The drawing under review shows one solid part. Ordinate dimensions are in mm from its lowest x, y, z. Coordinates: 2 decimals unless noted, no trailing zeros. Write each loop counter-clockwise with the first axis right and the second up, starting at its lowest first coordinate (ties: lowest second). Pieces come first, ordered by that corner, then holes. Notation, with made-up numbers: (61, -30.75) - (93, -30.75) arc R9 cw to (93, -15.75) - close; hole circle Ø10 at (7.25, 71). An arc over 180 degrees is marked (long way). Use a Markdown table: item, result.
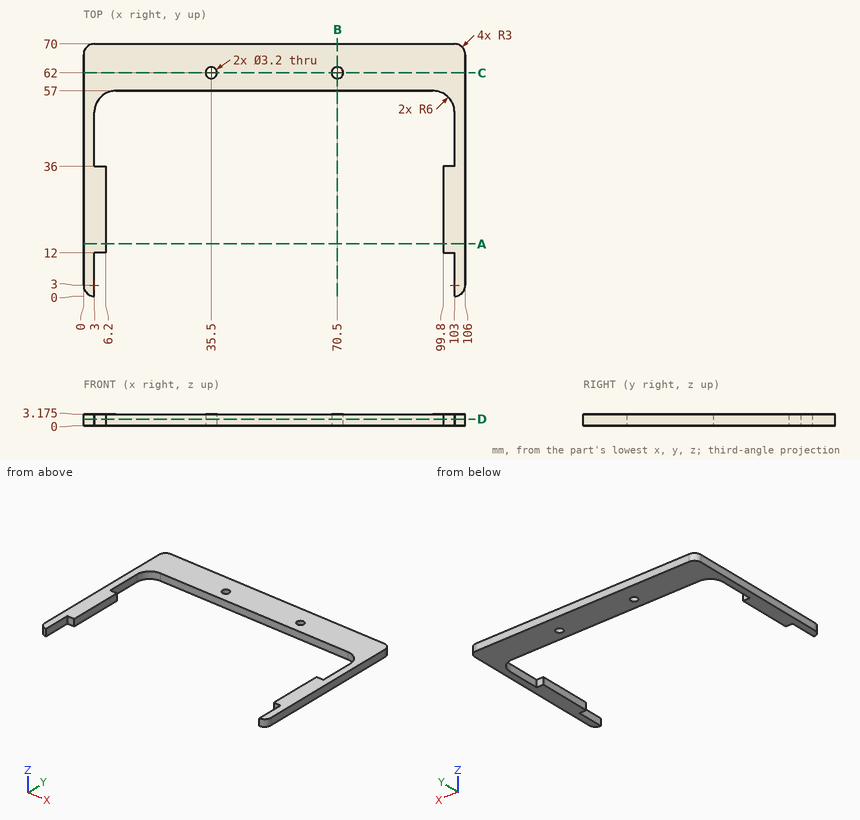
(1) Take a section at A-A on y = 14.5. Write out the cut boundary in (x, z) (3 decimals), and give its area (3 significant figures).
Determined:
| item | result |
|---|---|
| outline | (0, 0) - (6.2, 0) - (6.2, 3.175) - (0, 3.175) - close; (99.8, 0) - (106, 0) - (106, 3.175) - (99.8, 3.175) - close |
| area | 39.4 mm2 |
(2) Take a section at C-C on y = 62. Write out the cut boundary in (x, z) (3 decimals).
Determined:
| item | result |
|---|---|
| outline | (0, 0) - (33.9, 0) - (33.9, 3.175) - (0, 3.175) - close; (37.1, 0) - (68.9, 0) - (68.9, 3.175) - (37.1, 3.175) - close; (72.1, 0) - (106, 0) - (106, 3.175) - (72.1, 3.175) - close |
(3) Take a section at D-D on z = 1.8. Write out the cut boundary in (x, y), and give its area (3 significant figures).
Determined:
| item | result |
|---|---|
| outline | (0, 3) arc R3 ccw to (3, 0) - (3, 12) - (6.2, 12) - (6.2, 36) - (3, 36) - (3, 51) arc R6 cw to (9, 57) - (97, 57) arc R6 cw to (103, 51) - (103, 36) - (99.8, 36) - (99.8, 12) - (103, 12) - (103, 0) arc R3 ccw to (106, 3) - (106, 67) arc R3 ccw to (103, 70) - (3, 70) arc R3 ccw to (0, 67) - close; hole circle Ø3.2 at (35.5, 62); hole circle Ø3.2 at (70.5, 62) |
| area | 1,870 mm2 |
(4) Take a section at B-B on x = 70.5. Write out the cut boundary in (y, z) (3 decimals).
Determined:
| item | result |
|---|---|
| outline | (57, 0) - (60.4, 0) - (60.4, 3.175) - (57, 3.175) - close; (63.6, 0) - (70, 0) - (70, 3.175) - (63.6, 3.175) - close |
(5) For L1, parallel to X at y = 63, z = 1.9; L2, parallel to X at y = 8, z = 0.65; L3, parallel to X at y = 35.5, z = 2.6, list the stretches that pass through material, from the lowest coordinate up. Write a range as from..to.
Determined:
| item | result |
|---|---|
| L1 | 0..34.25, 36.75..69.25, 71.75..106 |
| L2 | 0..3, 103..106 |
| L3 | 0..6.2, 99.8..106 |
(6) For pin 1 (1.6 mm diameter, centred on x = 4.5, z = 1.5, fed in from -Y); pin 2 (1.6 mm diameter, centred on x = 62.5, z = 1, fed in from -Y); pin 3 (3 mm diameter, centred on x = 70.5, y = 62, fed in from -Z), all flat-tipped, find the tip position at first contact; note any pin that passes through.
Determined:
| item | result |
|---|---|
| pin 1 | y = 12 |
| pin 2 | y = 57 |
| pin 3 | through |
